Here's how the part is built. I have some questions about the finished solid (model axes, mm). A direction names the side the tool comes from. Round coordinates to 2 decimals unless told otherwise and drop trailing zeros. Write each loop counter-clockwise with the first axis right and the second up, starting at its lowest first coordinate (ties: lowest second). Pieces come first, ordered by that corner, then holes. Notation, with made-up numbers: M 15,76.25 L 29,76.25 A16 ccw 29,105.25 Z; hole C -16,18.25 d11. An arc over 180 degrees is marked long. Use one line per item in the form item = value. Start each with the question number.
Q1. I need wall thicknesses on line 1 along X through (y, z) = (-5.75, 0.3); line 2 along X through (y, z) = (-1, -0.1); line 3 along Y through (x, z) = (-3, 1.85). Which ranges of each line are inside material? Lowest first, please. Write a range as from..to.
Q2. I'm going to push flat-ended pins straight in: pin 1 Ø1 at (x, y) = (-3.5, -2.5) entering from -Z; pin 2 Ø1 at (x, y) = (-8, -3.5) entering from +Z; pin 3 Ø1.3 at (x, z) = (-9.5, 0.5) entering from -Y. Where does each tip first touch, or does it pass through?
Q3. We'd pull the mould along X, two halves only. Please class faces 1 (the face through (-9.656, 6.681, 1.252)), 2 (the face through (2.49, -8.04, 1.25)), 3 (the face through (-0.047, -3.047, -0.157)): +X half, -X half, draft (parallel to the pull), parting line (faces both ways), or undercut.
Q4. For faces 4 (the face through (0.047, 3.047, 2.697)), 5 (the face through (7.719, 6.076, 1.252)), which set-ups out of +Z, -Z, +X, -X, +Y, -Y let a thin tool reach every point of the face, with its end or its side?
Q5. I want a section at C-C on z = 1. State how many separate pieces and enclosed holes the cut face has, and give its area (3 significant figures).
Q6. I want a section at B-B on y = 0. List the corners of the cut face in (x, z) for me, and give its area (3 significant figures).
Q7. I want a section at A-A on x = 0. List the corners of the cut face in (y, z) for me.
Q8. I want a section at D-D on y = -4. List the corners of the cut face in (x, z) for me.
```python
from build123d import *

# Parameters (mm, degrees)
SKETCH1_R           = 12.8778
BOSS_EXTRUDE1_DEPTH = 2.54
BOSS_EXTRUDE2_DEPTH = 0.3175


with BuildPart() as part:
    # Sketch1 → Boss-Extrude1 (new body)
    with BuildSketch(Plane.XY):
        Circle(SKETCH1_R)
        with BuildLine():
            Line((1.8415, 0.889), (1.8415, -0.889))
            ThreePointArc((1.8415, -0.889), (0, -2.7305), (-1.8415, -0.889))
            Line((-1.8415, -0.889), (-1.8415, 0.889))
            ThreePointArc((-1.8415, 0.889), (0, 2.7305), (1.8415, 0.889))
        make_face(mode=Mode.SUBTRACT)
        with BuildLine():
            Line((0.635, 10.9728), (0.635, 8.4328))
            ThreePointArc((0.635, 8.4328), (0, 7.7978), (-0.635, 8.4328))
            Line((-0.635, 8.4328), (-0.635, 10.9728))
            ThreePointArc((-0.635, 10.9728), (0, 11.6078), (0.635, 10.9728))
        make_face(mode=Mode.SUBTRACT)
        with BuildLine():
            Line((4.092815459, 10.223987594), (3.307912294, 7.808304043))
            ThreePointArc((3.307912294, 7.808304043), (2.507765614, 7.400608947), (2.100070518, 8.200755626))
            Line((2.100070518, 8.200755626), (2.884973684, 10.616439177))
            ThreePointArc((2.884973684, 10.616439177), (3.685120363, 11.024134274), (4.092815459, 10.223987594))
        make_face(mode=Mode.SUBTRACT)
        with BuildLine():
            Line((7.149997625, 8.443300936), (5.657023085, 6.388397771))
            ThreePointArc((5.657023085, 6.388397771), (4.770053658, 6.247915614), (4.629571502, 7.134885041))
            Line((4.629571502, 7.134885041), (6.122546043, 9.189788207))
            ThreePointArc((6.122546043, 9.189788207), (7.009515469, 9.330270363), (7.149997625, 8.443300936))
        make_face(mode=Mode.SUBTRACT)
        with BuildLine():
            Line((9.507288207, 5.805046043), (7.452385041, 4.312071502))
            ThreePointArc((7.452385041, 4.312071502), (6.565415614, 4.452553658), (6.705897771, 5.339523085))
            Line((6.705897771, 5.339523085), (8.760800936, 6.832497625))
            ThreePointArc((8.760800936, 6.832497625), (9.647770363, 6.692015469), (9.507288207, 5.805046043))
        make_face(mode=Mode.SUBTRACT)
        with BuildLine():
            Line((10.933939177, 2.567473684), (8.518255626, 1.782570518))
            ThreePointArc((8.518255626, 1.782570518), (7.718108947, 2.190265614), (8.125804043, 2.990412294))
            Line((8.125804043, 2.990412294), (10.541487594, 3.775315459))
            ThreePointArc((10.541487594, 3.775315459), (11.341634274, 3.367620363), (10.933939177, 2.567473684))
        make_face(mode=Mode.SUBTRACT)
        with BuildLine():
            Line((11.2903, -0.9525), (8.7503, -0.9525))
            ThreePointArc((8.7503, -0.9525), (8.1153, -0.3175), (8.7503, 0.3175))
            Line((8.7503, 0.3175), (11.2903, 0.3175))
            ThreePointArc((11.2903, 0.3175), (11.9253, -0.3175), (11.2903, -0.9525))
        make_face(mode=Mode.SUBTRACT)
        with BuildLine():
            Line((10.541487594, -4.410315459), (8.125804043, -3.625412294))
            ThreePointArc((8.125804043, -3.625412294), (7.718108947, -2.825265614), (8.518255626, -2.417570518))
            Line((8.518255626, -2.417570518), (10.933939177, -3.202473684))
            ThreePointArc((10.933939177, -3.202473684), (11.341634274, -4.002620363), (10.541487594, -4.410315459))
        make_face(mode=Mode.SUBTRACT)
        with BuildLine():
            Line((8.760800936, -7.467497625), (6.705897771, -5.974523085))
            ThreePointArc((6.705897771, -5.974523085), (6.565415614, -5.087553658), (7.452385041, -4.947071502))
            Line((7.452385041, -4.947071502), (9.507288207, -6.440046043))
            ThreePointArc((9.507288207, -6.440046043), (9.647770363, -7.327015469), (8.760800936, -7.467497625))
        make_face(mode=Mode.SUBTRACT)
        with BuildLine():
            Line((6.122546043, -9.824788207), (4.629571502, -7.769885041))
            ThreePointArc((4.629571502, -7.769885041), (4.770053658, -6.882915614), (5.657023085, -7.023397771))
            Line((5.657023085, -7.023397771), (7.149997625, -9.078300936))
            ThreePointArc((7.149997625, -9.078300936), (7.009515469, -9.965270363), (6.122546043, -9.824788207))
        make_face(mode=Mode.SUBTRACT)
        with BuildLine():
            Line((2.884973684, -11.251439177), (2.100070518, -8.835755626))
            ThreePointArc((2.100070518, -8.835755626), (2.507765614, -8.035608947), (3.307912294, -8.443304043))
            Line((3.307912294, -8.443304043), (4.092815459, -10.858987594))
            ThreePointArc((4.092815459, -10.858987594), (3.685120363, -11.659134274), (2.884973684, -11.251439177))
        make_face(mode=Mode.SUBTRACT)
        with BuildLine():
            Line((-0.635, -11.6078), (-0.635, -9.0678))
            ThreePointArc((-0.635, -9.0678), (0, -8.4328), (0.635, -9.0678))
            Line((0.635, -9.0678), (0.635, -11.6078))
            ThreePointArc((0.635, -11.6078), (0, -12.2428), (-0.635, -11.6078))
        make_face(mode=Mode.SUBTRACT)
        with BuildLine():
            Line((-4.092815459, -10.858987594), (-3.307912294, -8.443304043))
            ThreePointArc((-3.307912294, -8.443304043), (-2.507765614, -8.035608947), (-2.100070518, -8.835755626))
            Line((-2.100070518, -8.835755626), (-2.884973684, -11.251439177))
            ThreePointArc((-2.884973684, -11.251439177), (-3.685120363, -11.659134274), (-4.092815459, -10.858987594))
        make_face(mode=Mode.SUBTRACT)
        with BuildLine():
            Line((-7.149997625, -9.078300936), (-5.657023085, -7.023397771))
            ThreePointArc((-5.657023085, -7.023397771), (-4.770053658, -6.882915614), (-4.629571502, -7.769885041))
            Line((-4.629571502, -7.769885041), (-6.122546043, -9.824788207))
            ThreePointArc((-6.122546043, -9.824788207), (-7.009515469, -9.965270363), (-7.149997625, -9.078300936))
        make_face(mode=Mode.SUBTRACT)
        with BuildLine():
            Line((-9.507288207, -6.440046043), (-7.452385041, -4.947071502))
            ThreePointArc((-7.452385041, -4.947071502), (-6.565415614, -5.087553658), (-6.705897771, -5.974523085))
            Line((-6.705897771, -5.974523085), (-8.760800936, -7.467497625))
            ThreePointArc((-8.760800936, -7.467497625), (-9.647770363, -7.327015469), (-9.507288207, -6.440046043))
        make_face(mode=Mode.SUBTRACT)
        with BuildLine():
            Line((-10.933939177, -3.202473684), (-8.518255626, -2.417570518))
            ThreePointArc((-8.518255626, -2.417570518), (-7.718108947, -2.825265614), (-8.125804043, -3.625412294))
            Line((-8.125804043, -3.625412294), (-10.541487594, -4.410315459))
            ThreePointArc((-10.541487594, -4.410315459), (-11.341634274, -4.002620363), (-10.933939177, -3.202473684))
        make_face(mode=Mode.SUBTRACT)
        with BuildLine():
            Line((-11.2903, 0.3175), (-8.7503, 0.3175))
            ThreePointArc((-8.7503, 0.3175), (-8.1153, -0.3175), (-8.7503, -0.9525))
            Line((-8.7503, -0.9525), (-11.2903, -0.9525))
            ThreePointArc((-11.2903, -0.9525), (-11.9253, -0.3175), (-11.2903, 0.3175))
        make_face(mode=Mode.SUBTRACT)
        with BuildLine():
            Line((-10.541487594, 3.775315459), (-8.125804043, 2.990412294))
            ThreePointArc((-8.125804043, 2.990412294), (-7.718108947, 2.190265614), (-8.518255626, 1.782570518))
            Line((-8.518255626, 1.782570518), (-10.933939177, 2.567473684))
            ThreePointArc((-10.933939177, 2.567473684), (-11.341634274, 3.367620363), (-10.541487594, 3.775315459))
        make_face(mode=Mode.SUBTRACT)
        with BuildLine():
            Line((-8.760800936, 6.832497625), (-6.705897771, 5.339523085))
            ThreePointArc((-6.705897771, 5.339523085), (-6.565415614, 4.452553658), (-7.452385041, 4.312071502))
            Line((-7.452385041, 4.312071502), (-9.507288207, 5.805046043))
            ThreePointArc((-9.507288207, 5.805046043), (-9.647770363, 6.692015469), (-8.760800936, 6.832497625))
        make_face(mode=Mode.SUBTRACT)
        with BuildLine():
            Line((-6.122546043, 9.189788207), (-4.629571502, 7.134885041))
            ThreePointArc((-4.629571502, 7.134885041), (-4.770053658, 6.247915614), (-5.657023085, 6.388397771))
            Line((-5.657023085, 6.388397771), (-7.149997625, 8.443300936))
            ThreePointArc((-7.149997625, 8.443300936), (-7.009515469, 9.330270363), (-6.122546043, 9.189788207))
        make_face(mode=Mode.SUBTRACT)
        with BuildLine():
            Line((-2.884973684, 10.616439177), (-2.100070518, 8.200755626))
            ThreePointArc((-2.100070518, 8.200755626), (-2.507765614, 7.400608947), (-3.307912294, 7.808304043))
            Line((-3.307912294, 7.808304043), (-4.092815459, 10.223987594))
            ThreePointArc((-4.092815459, 10.223987594), (-3.685120363, 11.024134274), (-2.884973684, 10.616439177))
        make_face(mode=Mode.SUBTRACT)
    extrude(amount=BOSS_EXTRUDE1_DEPTH)

    # Sketch2 → Boss-Extrude2 (add)
    with BuildSketch(Plane.XY.offset(2.54)):
        with BuildLine():
            Line((-2.159, 0.889), (-2.159, -0.889))
            ThreePointArc((-2.159, -0.889), (0, -3.048), (2.159, -0.889))
            Line((2.159, -0.889), (2.159, 0.889))
            ThreePointArc((2.159, 0.889), (0, 3.048), (-2.159, 0.889))
        make_face()
        with BuildLine():
            Line((1.8415, -0.889), (1.8415, 0.889))
            ThreePointArc((1.8415, 0.889), (0, 2.7305), (-1.8415, 0.889))
            Line((-1.8415, 0.889), (-1.8415, -0.889))
            ThreePointArc((-1.8415, -0.889), (0, -2.7305), (1.8415, -0.889))
        make_face(mode=Mode.SUBTRACT)
    boss_extrude2 = extrude(amount=BOSS_EXTRUDE2_DEPTH)

    # Mirror1: Boss-Extrude2 across plane
    add(boss_extrude2.mirror(Plane.XY.offset(1.27)))


solid = part.part
```
Reported:
q1.line_1 = -11.52..-8.56, -6.51..6.51, 8.56..11.52
q1.line_2 = -2.16..-1.84, 1.84..2.16
q1.line_3 = -12.52..-11.46, -8.08..7.44, 10.83..12.52
q2.pin_1 = 0
q2.pin_2 = 2.54
q2.pin_3 = -9.35
q3.face_1 = undercut
q3.face_2 = undercut
q3.face_3 = parting line
q4.face_4 = +Z, +Y
q4.face_5 = +Z, -Z
q5.separate_pieces = 1
q5.enclosed_holes = 21
q5.area = 414 mm^2
q6.outline = M -12.88,0 L -11.84,0 L -11.84,2.54 L -12.88,2.54 Z; M -8.2,0 L -2.16,0 L -2.16,-0.32 L -1.84,-0.32 L -1.84,2.86 L -2.16,2.86 L -2.16,2.54 L -8.2,2.54 Z; M 1.84,-0.32 L 2.16,-0.32 L 2.16,0 L 8.2,0 L 8.2,2.54 L 2.16,2.54 L 2.16,2.86 L 1.84,2.86 Z; M 11.84,0 L 12.88,0 L 12.88,2.54 L 11.84,2.54 Z
q6.area = 38.0 mm^2
q7.outline = M -12.88,0 L -12.24,0 L -12.24,2.54 L -12.88,2.54 Z; M -8.43,0 L -3.05,0 L -3.05,-0.32 L -2.73,-0.32 L -2.73,2.86 L -3.05,2.86 L -3.05,2.54 L -8.43,2.54 Z; M 2.73,-0.32 L 3.05,-0.32 L 3.05,0 L 7.8,0 L 7.8,2.54 L 3.05,2.54 L 3.05,2.86 L 2.73,2.86 Z; M 11.61,0 L 12.88,0 L 12.88,2.54 L 11.61,2.54 Z
q8.outline = M -12.24,0 L -11.34,0 L -11.34,2.54 L -12.24,2.54 Z; M -9.28,0 L 9.28,0 L 9.28,2.54 L -9.28,2.54 Z; M 11.34,0 L 12.24,0 L 12.24,2.54 L 11.34,2.54 Z
